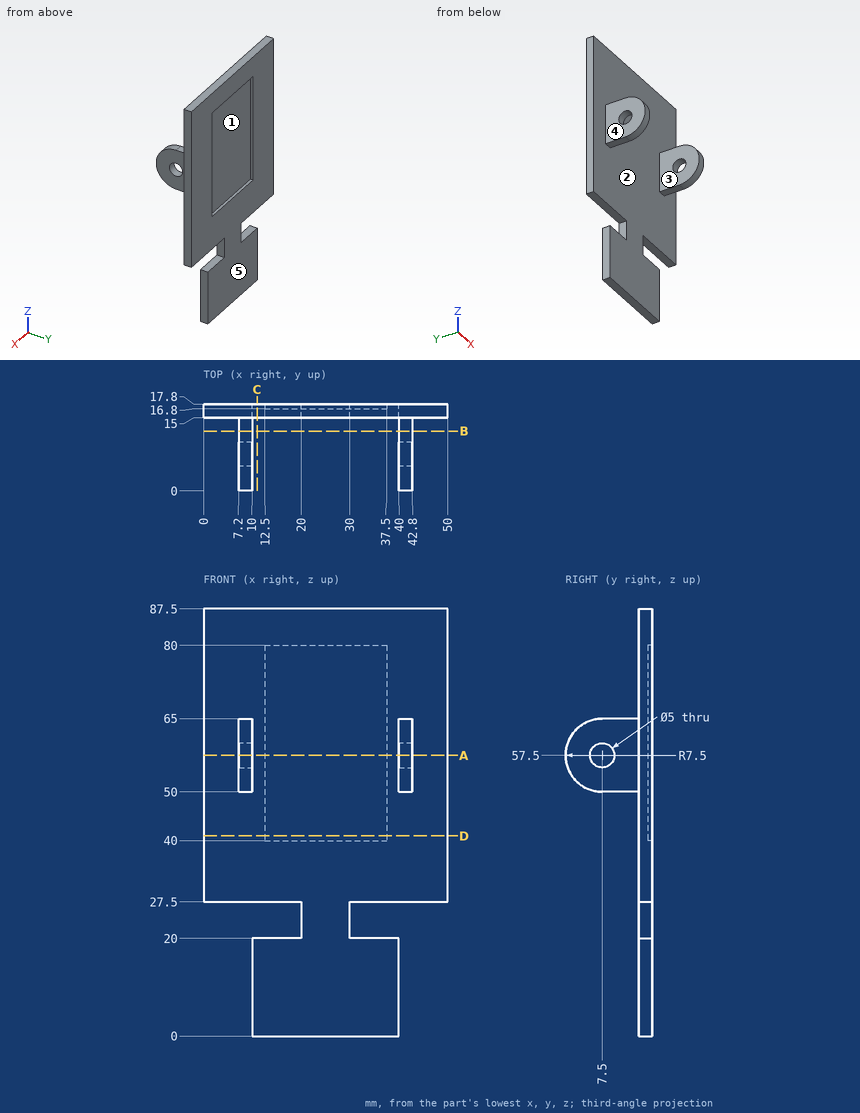
Geometry: see drawing. Coordinates: mm, zero at the bounding-box minimum. A direction names the side the tool comes from. Round coordinates to 2 decimals unless told otherwise and drop trailing zeros. Write each loop counter-clockwise with the first axis right and the second up, starting at its lowest first coordinate (ties: lowest second). Pieces come first, ordered by that corner, then holes.
Item 1: Section query B-B (y = 12.25). Return loops of the section in (x, z).
Item 2: Material intervals for L1, parallel to Z at x = 40.8, y = 7.5; L2, parallel to Y at x = 8.5, z = 57.5; L3, parallel to X at y = 11, z = 63.5, sorted ascending.
Item 3: Mould query, pull axis Z, two halves, no side actions, for the marked faces 1 and 2. Classes: +Z half, -Z half, draft (parallel to the pull), parting line (faces both ways), or undercut.
Item 4: Section query C-C (x = 11). Return loops of the section in (y, z).
Item 5: Set-up query: the marked faces 3, 4 and 5. Return all of +Z, -Z, +X, -X, +Y, -Y with unobstructed straight access to the full face (end or side cutting, diameter ignored); none if empty.
Item 6: Section query D-D (z = 41). Return loops of the section in (x, y), plus the area to 3 significant figures.
Item 7: Section query A-A (z = 57.5). Return loops of the section in (x, y).
Item 8: Pin query (flat end, axial travel): P1, Ø8, axis at y = 7.5, z = 57.5, coming from the +X side; P2, Ø2, axis at y = 16, z = 14, coming from the -X side; P3, Ø2, axis at x = 9, y = 13, coming from the -Z side; P4, Ø8, axis at x = 33.5, y = 10, coming from the +Z side. Return the tip coordinate at first contact, or that it passes through.
Completed:
1. outline: (7.2, 50) - (10, 50) - (10, 65) - (7.2, 65) - close; (40, 50) - (42.8, 50) - (42.8, 65) - (40, 65) - close
2. L1: z = 50 to 55, 60 to 65
2. L2: y = 0 to 5, 10 to 17.8
2. L3: x = 7.2 to 10, 40 to 42.8
3. face 1: undercut
3. face 2: draft
4. outline: (15, 0) - (17.8, 0) - (17.8, 20) - (15, 20) - close; (15, 27.5) - (17.8, 27.5) - (17.8, 87.5) - (15, 87.5) - close
5. face 3: +Z, -Z, -Y
5. face 4: +Z, -Z, -X, -Y
5. face 5: +Z, -Z, +X, -X, +Y
6. outline: (0, 15) - (50, 15) - (50, 17.8) - (37.5, 17.8) - (37.5, 16.8) - (12.5, 16.8) - (12.5, 17.8) - (0, 17.8) - close
6. area: 115 mm2
7. outline: (0, 15) - (7.2, 15) - (7.2, 10) - (10, 10) - (10, 15) - (40, 15) - (40, 10) - (42.8, 10) - (42.8, 15) - (50, 15) - (50, 17.8) - (37.5, 17.8) - (37.5, 16.8) - (12.5, 16.8) - (12.5, 17.8) - (0, 17.8) - close; (7.2, 0) - (10, 0) - (10, 5) - (7.2, 5) - close; (40, 0) - (42.8, 0) - (42.8, 5) - (40, 5) - close
8. P1: stops at x = 42.8
8. P2: stops at x = 10
8. P3: stops at z = 50
8. P4: passes through
